```python
from build123d import *

# Parameters (mm, degrees)
SKETCH1_W           = 120
SKETCH1_H           = 79
SKETCH1_W_2         = 25.82
SKETCH1_H_2         = 3
BOSS_EXTRUDE1_DEPTH = 3


with BuildPart() as part:
    # Sketch1 → Boss-Extrude1 (new body)
    with BuildSketch(Plane.XY):
        Polygon((-68, 0), (65, 0), (65, -43.007142857), (68, -43.007142857), (68, -85.714285714), (65, -85.714285714), (65, -128.721428571), (68, -128.721428571), (68, -171.428571429), (65, -171.428571429), (65, -214.435714286), (68, -214.435714286), (68, -257.142857143), (65, -257.142857143), (65, -300.15), (68, -300.15), (68, -342.857142857), (65, -342.857142857), (65, -385.864285714), (68, -385.864285714), (68, -428.571428571), (65, -428.571428571), (65, -471.578571429), (68, -471.578571429), (68, -514.285714286), (65, -514.285714286), (65, -557.292857143), (68, -557.292857143), (68, -600), (-65, -600), (-65, -557.292857143), (-68, -557.292857143), (-68, -514.285714286), (-65, -514.285714286), (-65, -471.578571429), (-68, -471.578571429), (-68, -428.571428571), (-65, -428.571428571), (-65, -385.864285714), (-68, -385.864285714), (-68, -342.857142857), (-65, -342.857142857), (-65, -300.15), (-68, -300.15), (-68, -257.142857143), (-65, -257.142857143), (-65, -214.435714286), (-68, -214.435714286), (-68, -171.428571429), (-65, -171.428571429), (-65, -128.721428571), (-68, -128.721428571), (-68, -85.714285714), (-65, -85.714285714), (-65, -43.007142857), (-68, -43.007142857), align=None)
        with Locations((0, -555.5)):
            Rectangle(SKETCH1_W, SKETCH1_H, mode=Mode.SUBTRACT)
        with Locations((-25.97, -151.5)):
            Rectangle(SKETCH1_W_2, SKETCH1_H_2, mode=Mode.SUBTRACT)
        with Locations((25.97, -151.5)):
            Rectangle(SKETCH1_W_2, SKETCH1_H_2, mode=Mode.SUBTRACT)
        with Locations((-25.97, -504.5)):
            Rectangle(SKETCH1_W_2, SKETCH1_H_2, mode=Mode.SUBTRACT)
        with Locations((25.97, -504.5)):
            Rectangle(SKETCH1_W_2, SKETCH1_H_2, mode=Mode.SUBTRACT)
    extrude(amount=BOSS_EXTRUDE1_DEPTH)


solid = part.part
```
Part model, mm, in its own coordinate system. Give positions to 0.01 mm unless a question says otherwise; leave off trailing zeros. Order: outer loops, then holes, each group sorted by start corner. A loop starts at its lowest first (then second) coordinate and runs counter-clockwise, first axis right, second up. Notation, with made-up numbers: M 30,-24.75 L 53,-24.75 A17 cw 53,5.25 Z; hole C -14.5,54 d5. An arc over 180 degrees is marked long. Use a Markdown table: item, result. Add a question column.
(1) Saw through at A-A, the plane x = 23. Give the cut face in (y, z), and give its area (4 significant figures).
(2) Saw through at B-B, the plane x = 46.5. Give the cut face in (y, z).
(3) Drop flat-ended pins along their axis: P1, Ø6, axis at x = 53, y = -397, coming from the -Z side; P2, Ø0.9, axis at x = 66.5, z = 1, coming from the +Y side; P3, Ø0.9, axis at x = -67, z = 1.5, coming from the -Y side; P4, Ø1.5, axis at y = -504, z = 1, coming from the -X side. Give the stop position or say it passes through.
(4) Probe line 1 along Y through (x, z) = (17, 0.2); line 2 along X through (y, z) = (-152, 1.6); line 3 along Y through (x, z) = (-4.5, 2.65). List the from-to ranges inside material, lowest first. Write a range as [from, to].
(5) Saw through at C-C, the plane z = 0.45. Give the number of separate pieces and of enclosed holes in the cut face, and give its area (3 significant figures).
(6) Saw through at D-D, the plane y = -234.5. Give the cut face in (x, z).
Answer key:
| question | item | result |
|---|---|---|
| 1 | outline | M -600,0 L -595,0 L -595,3 L -600,3 Z; M -516,0 L -506,0 L -506,3 L -516,3 Z; M -503,0 L -153,0 L -153,3 L -503,3 Z; M -150,0 L 0,0 L 0,3 L -150,3 Z |
| 1 | area | 1,545 mm^2 |
| 2 | outline | M -600,0 L -595,0 L -595,3 L -600,3 Z; M -516,0 L 0,0 L 0,3 L -516,3 Z |
| 3 | P1 | z = 0 |
| 3 | P2 | y = -43.01 |
| 3 | P3 | y = -557.29 |
| 3 | P4 | x = -65 |
| 4 | line 1 | [-600, -595], [-516, -506], [-503, -153], [-150, 0] |
| 4 | line 2 | [-65, -38.88], [-13.06, 13.06], [38.88, 68] |
| 4 | line 3 | [-600, -595], [-516, 0] |
| 5 | separate pieces | 1 |
| 5 | enclosed holes | 5 |
| 5 | area | 70,000 mm^2 |
| 6 | outline | M -65,0 L 68,0 L 68,3 L -65,3 Z |
